Geometry: final body of the model. Coordinates: model frame, mm. Face numbers are marked on the shaded views. A direction names the side the tool comes from. Give positions to 0.01 mm unless a question says otherwise; leave off trailing zeros. Loops run counter-clockwise (first coordinate to the right, second up) from the corner with the lowest first, then second, coordinate; pieces in that order, holes last. Notation, with made-up numbers: (41, 89.25) -> (69, 89.25) arc R20 ccw to (69, 124.25) -> close; hole circle Ø2 at (27.5, 45). An arc over 180 degrees is marked (long way). Answer in a Markdown table with one row per item. Add a question column.
1) Access query for the marked faces 4 and 5. Directions: +Z, -Z, +X, -X, +Y, -Y. A direction counts if a zero-diameter tool reaches every point of the face in a straight line with its end or side. Return the directions, or none.
2) Section query B-B (z = 0). Return the cut outline in (x, y) (1 decimal).
3) Section query C-C (x = -8.25). Return the cut outline in (y, z) (1 decimal).
4) Section query A-A (y = 0). Return the cut outline in (x, z), plus the area to 3 significant figures.
5) Line query: line 1 (Z direction, x = -8.5, y = 0); line 2 (Y direction, x = -16, z = 0); line 3 (Y direction, x = -9.25, z = 0). Output: solid intervals per line, ascending. Write a range as from..to.
6) First-contact query: P1, Ø2, axis at x = -18.5, z = -5.5, coming from the -Y side; P2, Ø1, axis at x = -8, z = -5.5, coming from the +Y side; P3, Ø3.5, axis at x = -15, z = 1, coming from the -Y side. Flat tips, straight axial feed; report the tip coordinate or a pass-through.
7) Draft query along Y for the marked faces 1, 2 and 3. Return one class per face: +Y half, -Y half, draft (parallel to the pull), parting line (faces both ways), or undercut.
```python
from build123d import *

# Parameters (mm, degrees)
F0_W           = 25.4
F0_H           = 25.4
F1_DEPTH       = 12.7
F3_D           = 9.525
F3_CSINK_D     = 10.795
F3_CSINK_ANGLE = 45
F5_R           = 3.175
F6_DEPTH       = 24.13


# Not quite as in the source:
# - a pattern or mirror of a feature is missing from the dataset's text; its kind, count and spacing are read off the source's solid


with BuildPart() as f1:
    # F0 (on Right) → F1 (new body)
    with BuildSketch(Plane.YZ):
        Rectangle(F0_W, F0_H)
    extrude(amount=-F1_DEPTH)

    # F3 (through all)
    with Locations(Plane.YZ):
        with Locations((0, 0)):
            CounterSinkHole(F3_D / 2, F3_CSINK_D / 2, counter_sink_angle=F3_CSINK_ANGLE)

    # F4: F1 across face


with BuildPart() as f1_1:
    add(f1.part)
    add(f1.part.mirror(Plane(origin=(-12.7, 0, 0), x_dir=(0, 1, 0), z_dir=(-1, 0, 0))))

    # F5 (on face) → F6 (join)
    with BuildSketch(Plane.XZ.offset(12.7)):
        with Locations((-12.7, 0)):
            Circle(F5_R)
    f6 = extrude(amount=F6_DEPTH)

    # F6_copies: F6 across plane
    add(f6.mirror(Plane.ZX))

    # F8 (on offset) → F9 (revolve)
    with BuildSketch(Plane(origin=(-12.7, 0, 0), x_dir=(0, -1, 0), z_dir=(-1, 0, 0))):
        with BuildLine():
            Line((36.83, 5.715), (36.83, 3.175))
            Line((36.83, 3.175), (36.83, 0))
            Line((36.83, 0), (42.545, 0))
            ThreePointArc((42.545, 0), (40.8711152545, 4.0411152545), (36.83, 5.715))
        make_face()
    f9 = revolve(axis=Axis((-12.7, -39.6875, 0), (0, 1, 0)))

    # F9_copies: F9 across plane
    add(f9.mirror(Plane.ZX))


solid = f1_1.part
```
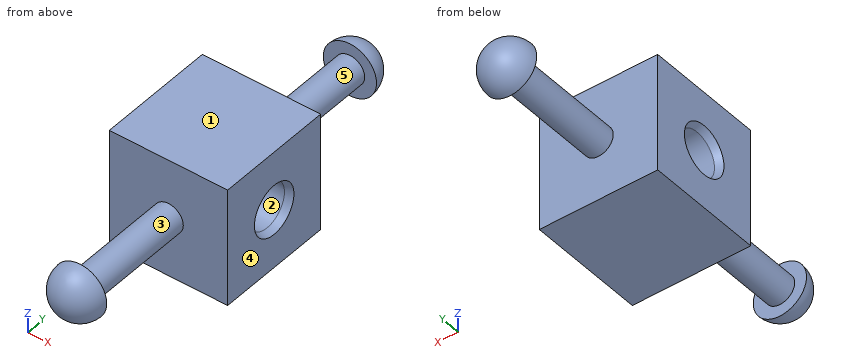
Evaluation:
| question | item | result |
|---|---|---|
| 1 | face 4 | +Z, -Z, +X, +Y, -Y |
| 1 | face 5 | none |
| 2 | outline | (-25.4, -12.7) -> (-15.9, -12.7) -> (-15.9, -36.8) -> (-18.4, -36.8) arc R5.7 ccw to (-7, -36.8) -> (-9.5, -36.8) -> (-9.5, -12.7) -> (0, -12.7) -> (0, -5.4) -> (-1.5, -4.8) -> (-23.9, -4.8) -> (-25.4, -5.4) -> close; (-25.4, 5.4) -> (-23.9, 4.8) -> (-1.5, 4.8) -> (0, 5.4) -> (0, 12.7) -> (-9.5, 12.7) -> (-9.5, 36.8) -> (-7, 36.8) arc R5.7 ccw to (-18.4, 36.8) -> (-15.9, 36.8) -> (-15.9, 12.7) -> (-25.4, 12.7) -> close |
| 3 | outline | (-36.8, -3.6) -> (-36.8, 3.6) arc R3.6 ccw to start; (-12.7, -12.7) -> (12.7, -12.7) -> (12.7, 12.7) -> (-12.7, 12.7) -> close; (36.8, -3.6) arc R3.6 ccw to (36.8, 3.6) -> close; hole circle Ø9.5 at (0, 0) |
| 4 | outline | (-25.4, -12.7) -> (0, -12.7) -> (0, -5.4) -> (-1.53, -4.76) -> (-23.87, -4.76) -> (-25.4, -5.4) -> close; (-25.4, 5.4) -> (-23.87, 4.76) -> (-1.53, 4.76) -> (0, 5.4) -> (0, 12.7) -> (-25.4, 12.7) -> close |
| 4 | area | 401 mm² |
| 5 | line 1 | -12.7..-4.76, 4.76..12.7 |
| 5 | line 2 | -41.5..-36.83, -12.7..-4.76, 4.76..12.7, 36.83..41.5 |
| 5 | line 3 | -41.39..-36.83, -12.7..-4.76, 4.76..12.7, 36.83..41.39 |
| 6 | P1 | y = -12.7 |
| 6 | P2 | y = 12.7 |
| 6 | P3 | y = -42.49 |
| 7 | face 1 | draft |
| 7 | face 2 | undercut |
| 7 | face 3 | undercut |
